from build123d import *

# Parameters (mm, degrees)
SKETCH2_R               = 11.25
SKETCH2_R_2             = 10.65
CUT_EXTRUDE1_DEPTH      = 1035.156510288
CUT_EXTRUDE1_DEPTH_BACK = 1035.156510288
SKETCH3_R               = 3.238231215


with BuildPart() as part:
    # Sweep1: sweep along a path in Sketch1
    with BuildLine(Plane.XY) as sweep1_path:
        Line((0, 0), (0, 290))
        ThreePointArc((0, 290), (23.431457505, 346.568542495), (80, 370))
        Line((80, 370), (870, 370))
        ThreePointArc((870, 370), (926.568542495, 346.568542495), (950, 290))
        Line((950, 290), (950, 0))
    # Sketch2 → Sweep1 (sweep)
    with BuildSketch(Plane(origin=(0, 0, 0), x_dir=(1, 0, 0), z_dir=(0, 1, 0))):
        Circle(SKETCH2_R)
        Circle(SKETCH2_R_2, mode=Mode.SUBTRACT)
    sweep(path=sweep1_path.line)

    # Sketch3 → Cut-Extrude1 (cut, two sides: drawn at the far end of the back side and taken through both)
    with BuildSketch(Plane(origin=(0, 0, 0), x_dir=(0, 0, -1), z_dir=(1, 0, 0)).offset(-CUT_EXTRUDE1_DEPTH_BACK)):
        with Locations((0, 12)):
            Circle(SKETCH3_R)
        with Locations((0, 47)):
            Circle(SKETCH3_R)
    extrude(amount=CUT_EXTRUDE1_DEPTH + CUT_EXTRUDE1_DEPTH_BACK, mode=Mode.SUBTRACT)


solid = part.part
Could you check a few things on this model? Use its own coordinates, in mm. A direction names the side the tool comes from. Coordinates: 2 decimals unless noted, no trailing zeros. Write each loop counter-clockwise with the first axis right and the second up, starting at its lowest first coordinate (ties: lowest second). Pieces come first, ordered by that corner, then holes. Notation, with made-up numbers: (89, 20.25) - (136, 20.25) arc R9 ccw to (136, 31.25) - close; hole circle Ø4 at (24, 15.5). An arc over 180 degrees is marked (long way). Write item = value, one per line.
1) Suppose I cut it at B-B on x = 753.5. Please give me the cut outline in (y, z), plus the area to 3 significant figures.
Result set:
outline = circle Ø22.5 at (370, 0); hole circle Ø21.3 at (370, 0)
area = 41.3 mm2
2) Suppose I cut it at A-A on y = 121. Please give me the cut outline in (x, z), plus the area to 3 significant figures.
Result set:
outline = circle Ø22.5 at (0, 0); circle Ø22.5 at (950, 0); hole circle Ø21.3 at (0, 0); hole circle Ø21.3 at (950, 0)
area = 82.6 mm2
3) Please list where these lines run through material, in increasing order: line 1 (X direction, y = 99.5, z = -0.25); line 2 (Y direction, x = 678, z = -0.5); line 3 (X direction, y = 154.5, z = -5.5). Write a range as [from, to].
Result set:
line_1 = [-11.25, -10.65], [10.65, 11.25], [938.75, 939.35], [960.65, 961.25]
line_2 = [358.76, 359.36], [380.64, 381.24]
line_3 = [-9.81, -9.12], [9.12, 9.81], [940.19, 940.88], [959.12, 959.81]
4) For faces 4 (the flat face through (-9, 0, 6)), 5 (the cylindrical face through (480.53, 380.64, -0.47)), 6 (the cylindrical face through (939.61, 142.97, 4.31)), which set-ups out of +Z, -Z, +X, -X, +Y, -Y let a thin tool reach every point of the face, with its end or its side?
Result set:
face_4 = +Z, -Z, +X, -X, -Y
face_5 = none
face_6 = -Y
5) Will these pins go through, and if not, where does the flat tip stop? pin 1 Ø2 at (x, z) = (402.5, 8) entering from +Y; pin 2 Ø12 at (y, z) = (283, 5) entering from -X; pin 3 Ø10 at (y, z) = (115.5, -7) entering from +X; pin 4 Ø8 at (y, z) = (153.5, 8) entering from +X.
Result set:
pin_1 = 378.81
pin_2 = -11.25
pin_3 = 961.07
pin_4 = 960.51
6) We'd pull the mould along Z, two halves only. Please class faces 1 (the cylindrical face through (10.158, 147.03, -3.199)), 2 (the cylindrical face through (5.19, 147.03, 9.98)), 3 (the flat face through (941, 0, -6)): +Z half, -Z half, draft (parallel to the pull), parting line (faces both ways), or undercut.
Result set:
face_1 = undercut
face_2 = parting line
face_3 = draft
